```python
from build123d import *

# Parameters (mm, degrees)
SKETCH1_R           = 9
BOSS_EXTRUDE1_DEPTH = 10
SKETCH2_R           = 6
CUT_EXTRUDE1_DEPTH  = 3
CUT_EXTRUDE2_DEPTH  = 17.186414056
CIRPATTERN1_COUNT   = 30


with BuildPart() as part:
    # Sketch1 → Boss-Extrude1 (new body)
    with BuildSketch(Plane.XY):
        Circle(SKETCH1_R)
    extrude(amount=BOSS_EXTRUDE1_DEPTH)

    # Sketch2 → Cut-Extrude1 (cut)
    with BuildSketch(Plane.XY.offset(10)):
        Circle(SKETCH2_R)
    extrude(amount=-CUT_EXTRUDE1_DEPTH, mode=Mode.SUBTRACT)

    # Sketch3 → Cut-Extrude2 (cut, through all)
    with BuildSketch(Plane.XY.offset(10)):
        with BuildLine():
            Line((-1.633345226, 10.785436843), (1.633345226, 10.785436843))
            Line((1.633345226, 10.785436843), (0.6, 8.994081534))
            Line((0.6, 8.994081534), (0.086621258, 8.104113968))
            ThreePointArc((0.086621258, 8.104113968), (0, 8.054081534), (-0.086621258, 8.104113968))
            Line((-0.086621258, 8.104113968), (-0.6, 8.994081534))
            Line((-0.6, 8.994081534), (-1.633345226, 10.785436843))
        make_face()
    cut_extrude2 = extrude(amount=-CUT_EXTRUDE2_DEPTH, mode=Mode.SUBTRACT)

    # CirPattern1: Cut-Extrude2 ×30 about axis
    cirpattern1_axis = Axis((0, 0, 0), (0, 0, 1))
    for i in range(1, CIRPATTERN1_COUNT):
        add(cut_extrude2.rotate(cirpattern1_axis, i * 360 / CIRPATTERN1_COUNT), mode=Mode.SUBTRACT)


solid = part.part
```
Geometry check sheet. Reference: the model listing, model coordinates, mm. A direction names the side the tool comes from. Coordinates: 2 decimals unless noted, no trailing zeros. Order: outer loops, then holes, each group sorted by start corner. A loop starts at its lowest first (then second) coordinate and runs counter-clockwise, first axis right, second up. Notation, with made-up numbers: (-37, 20) - (-4, 20) arc R23 ccw to (-4, 32) - close; hole circle Ø6 at (-7, 25). An arc over 180 degrees is marked (long way). Answer in a Markdown table with one row per item. Add a question column.
1. Gauge pin test, flat ends, axial feed: pin 1 Ø0.8 at (x, z) = (7.5, 6.5) entering from -Y; pin 2 Ø1.5 at (x, y) = (1.5, -2.5) entering from -Z; pin 3 Ø1 at (y, z) = (2.5, 2.5) entering from +X; pin 4 Ø1.1 at (x, z) = (7.5, 6.5) entering from +Y. Record the tip position at first contact, or that the pin passes through.
2. Section check A-A (y = 0). Enter the section's corners in (x, z), plus the area to 3 significant figures.
3. Material ranges on L1, parallel to Y at x = -7, z = 3; L2, parallel to X at y = 6.75, z = 5.5; L3, parallel to Y at x = 0, z = 9.15, recorded low to high. Write a range as [from, to].
4. Draft check along Y on faces 1 (the face through (-8.54, -0.55, 5.07)), 2 (the face through (1.442, -8.433, 5.07)), 3 (the face through (3.79, 7.67, 5.07)). Enter one of: +Y half, -Y half, draft (parallel to the pull), parting line (faces both ways), or undercut.
5. Access from +Z, -Z, +X, -X, +Y, -Y to the whole of each face (thin tool, end or side, straight path). Record for faces 4 (the face through (-8.52, 0.56, 5.07)), 5 (the face through (-3.78, 7.66, 5.07)), 6 (the face through (7.225, 4.559, 5.07)), 7 (the face through (-1.446, -8.419, 5.07)), 8 (the face through (-6.582, -5.465, 5.07)).
Data:
| question | item | result |
|---|---|---|
| 1 | pin 1 | stops at y = -5.53 |
| 1 | pin 2 | stops at z = 0 |
| 1 | pin 3 | stops at x = 8.77 |
| 1 | pin 4 | stops at y = 5.57 |
| 2 | outline | (-9, 0) - (9, 0) - (9, 10) - (6, 10) - (6, 7) - (-6, 7) - (-6, 10) - (-9, 10) - close |
| 2 | area | 144 mm² |
| 3 | L1 | y = [-5.55, -4.17], [-4, 4], [4.17, 5.55] |
| 3 | L2 | x = [-5.95, -5.38], [-4.71, 4.71], [5.38, 5.95] |
| 3 | L3 | y = [-8.05, -6], [6, 8.05] |
| 4 | face 1 | undercut |
| 4 | face 2 | -Y half |
| 4 | face 3 | +Y half |
| 5 | face 4 | +Z, -Z, -X |
| 5 | face 5 | +Z, -Z, +Y |
| 5 | face 6 | +Z, -Z, +X |
| 5 | face 7 | +Z, -Z, -Y |
| 5 | face 8 | +Z, -Z |
